Job drawing, mm, ordinate dimensions from the low corner. One solid piece. A direction names the side the tool comes from. Round coordinates to 2 decimals unless told otherwise and drop trailing zeros. Loops run counter-clockwise (first coordinate to the right, second up) from the corner with the lowest first, then second, coordinate; pieces in that order, holes last. Notation, with made-up numbers: M -4.75,60 L 24.25,60 A8 cw 24.25,70 Z; hole C 52.25,-17 d9. An arc over 180 degrees is marked long. Write each question's results on one line, items separated by ' | '. Start each with the question number.
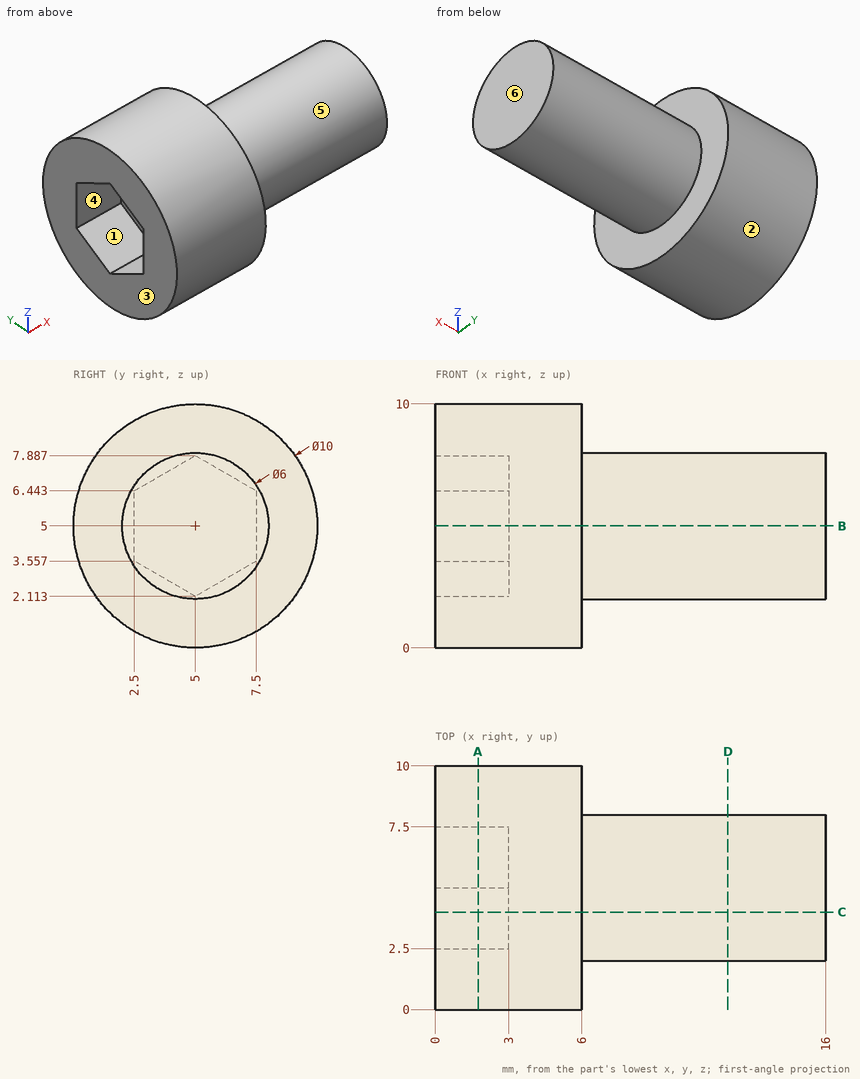
Item 1: Saw through at A-A, the plane x = 1.75. Give the cut face in (y, z).
Item 2: Saw through at B-B, the plane z = 5. Give the cut face in (x, y).
Item 3: Saw through at C-C, the plane y = 4. Give the cut face in (x, z).
Item 4: Mould opens along Y. For the marked faces 1, 2 and 3 say: released by +Y, released by -Y, zero draft, split by the parting line, or undercut.
Item 5: Saw through at D-D, the plane x = 12. Give the cut face in (y, z).
Item 6: Drill centre lines: line 1 along X through (y, z) = (3.5, 2.25); line 2 along X through (y, z) = (5, 5.75); line 3 along Y through (x, z) = (2.5, 2.5). Where is each one in solid material? Low to high. Write a range as [from, to].
Item 7: Drop flat-ended pins along their axis: pin 1 (1.5 mm diameter, centred on y = 4, z = 5, fed in from -X); pin 2 (6 mm diameter, centred on x = 13.5, y = 5, fed in from -Z); pin 3 (6 mm diameter, centred on x = 13, y = 8, fed in from +Z). Give the stop position or say it passes through.
Item 8: Tool access for the marked faces 4, 5 and 6: list every direction of +Z, -Z, +X, -X, +Y, -Y with a clear straight run to the whole face (end or side of a thin tool).
Working result:
1) outline: C 5,5 d10; hole M 2.5,3.56 L 5,2.11 L 7.5,3.56 L 7.5,6.44 L 5,7.89 L 2.5,6.44 Z
2) outline: M 0,0 L 6,0 L 6,2 L 16,2 L 16,8 L 6,8 L 6,10 L 0,10 L 0,7.5 L 3,7.5 L 3,2.5 L 0,2.5 Z
3) outline: M 0,0.1 L 6,0.1 L 6,2.17 L 16,2.17 L 16,7.83 L 6,7.83 L 6,9.9 L 0,9.9 L 0,7.31 L 3,7.31 L 3,2.69 L 0,2.69 Z
4) face 1: undercut | face 2: split by the parting line | face 3: zero draft
5) outline: C 5,5 d6
6) line 1: x = [0, 6] | line 2: x = [3, 16] | line 3: y = [0.67, 4.33], [5.67, 9.33]
7) pin 1: stops at x = 3 | pin 2: stops at z = 2 | pin 3: stops at z = 8
8) face 4: -X | face 5: +X | face 6: +Z, -Z, +X, +Y, -Y
